Autodesk Inventor part; units mm, degrees
ref_plane "YZ Plane" through (0, 0, 0) normal (1, 0, 0) x (0, 1, 0)
ref_plane "XZ Plane" through (0, 0, 0) normal (0, 1, 0) x (-1, 0, 0)
ref_plane "XY Plane" through (0, 0, 0) normal (0, 0, 1) x (1, 0, 0)
sketch "Sketch1" plane through (0, 0, 0) normal (0, 1, 0) x (-1, 0, 0)
  line L0 (0, 780) -> (0, 0)
  line L1 (727.158, 778) -> (727.158, 780)
  line L2 (727.158, 780) -> (0, 780)
  line L3 (727.158, 778) -> (110, 0)
  line L4 (110, 0) -> (0, 0)
  point P0 (0, 678)
  dimension "d1" = 727.158
  dimension "d2" = 2
  dimension "d5" = 128.424
  dimension "d6" = 110
  dimension "d9" = 780
extrude "Plate1" add sketch "Sketch1" along normal blind 3
mirror "Mirror1" about plane through (0, 0, 0) normal (1, 0, 0)
sketch "Sketch2" plane through (0, 0, 0) normal (0, -1, 0) x (1, 0, 0)
  line L0 (-110, 0) -> (110, 0) construction
  line L1 (-110, 0) -> (-727.158, 778) construction
  circle A0 centre (-325, 450) radius 84.5
  line L2 (110, 0) -> (727.158, 778) construction
  circle A1 centre (100, 450) radius 84.5
  circle A2 centre (410, 600) radius 45
  line L3 (-110, 0) -> (110, 0) construction
  line L4 (-240.5, 450) -> (-240.5, 164.5105) construction
  line L5 (365, 600) -> (365, 0) construction
  line L6 (-325, 534.5) -> (365, 534.5) construction
  line L7 (-325, 365.5) -> (365, 365.5) construction
  line L8 (100, 534.5) -> (365, 534.5) construction
  line L9 (410, 555) -> (365, 555) construction
  line L10 (-727.158, 780) -> (727.158, 780)
  line L11 (-727.158, 778) -> (-727.158, 780)
  line L12 (727.158, 778) -> (727.158, 780)
  point P0 (0, 0)
  point P1 (0, 0)
  point P2 (0, 0)
  point P3 (0, 0)
  point P4 (0, 0)
  point P5 (0, 0)
  point P6 (0, 0)
  dimension "d13" = 169
  dimension "d16" = 450
  dimension "d17" = 450
  dimension "d18" = 325
  dimension "d19" = -169
  dimension "d20" = 90
  dimension "d23" = 410
  dimension "d24" = 600
  dimension "d29" = 100
extrude "Extrusion1" cut sketch "Sketch2" against normal through all
sketch "Sketch3" plane through (0, 0, 0) normal (0, -1, 0) x (1, 0, 0)
  line L0 (-53.9958, 701.8167) -> (-53.9958, 713.8167) construction
  line L1 (-53.9958, 713.8167) -> (56.0042, 713.8167) construction
  line L2 (56.0042, 713.8167) -> (56.0042, 701.8167) construction
  line L3 (56.0042, 701.8167) -> (-53.9958, 701.8167) construction
  point P0 (0, 0)
  point P1 (1.0042, 701.8167)
  dimension "d25" = 12
  dimension "d26" = 110
mark "Mark1"
equation "\"d3\" = Thickness"
properties part number "MSC 701 FACE 1" material "Stainless Steel"
The listing builds one solid part. Answer for the finished solid, in the listing's coordinates (mm). Round coordinates to 2 decimals unless told otherwise and drop trailing zeros. Write each loop counter-clockwise with the first axis right and the second up, starting at its lowest first coordinate (ties: lowest second). Pieces come first, ordered by that corner, then holes. Notation, with made-up numbers: (-34.5, 38.25) -> (-26.5, 38.25) arc R12 ccw to (-26.5, 47.25) -> close; hole circle Ø8 at (37, 76). An arc over 180 degrees is marked (long way). Answer as a JSON object with one key per item and string values. Group by question number.
Q1. This flat-tipped pin is pushed along its axis until it touches: pin 1 Ø1 at (x, y) = (461, 2) entering from -Z. Where does it stop, or does it pass through?
Q2. Straight lines are drawn through the part: line 1 along X through (y, z) = (0.1, 498); line 2 along Z through (x, y) = (178, 1.95); line 3 along Z through (x, y) = (-325, 1.6). For each, find the intervals that lie inside material, in ascending order.
Q3. Section D-D (z = 450) is taken. Write down the section's boundary in (x, y).
Q4. Section A-A (z = 619) is taken. Write down the section's boundary in (x, y), plus the area to 3 significant figures.
Q5. Section C-C (y = 2.3) is taken. Write down the section's boundary in (x, z), plus the area to 3 significant figures.
Q6. Section B-B (x = -325) is taken. Write down the section's boundary in (y, z), plus the area to 3 significant figures.
Q7. Determine the mould class of faces 1 (the face through (434.192, 1.479, 637.944)), 2 (the face through (10, 3, 482)), 3 (the face through (-246.94, 1.48, 417.64)), 4 (the face through (414.259, 1.479, 383.554)) for opening direction Z: pulls with the +Z half, pulls with the -Z half, needs draft (parallel to the pull), parting line crosses it, or undercut.
Check values:
{
 "1": {"pin 1": "z = 441.85"},
 "2": {"line 1": "-505.04 to -394.54, -255.46 to 30.46, 169.54 to 505.04", "line 2": "85.72 to 417.5, 482.5 to 780", "line 3": "271.03 to 365.5, 534.5 to 780"},
 "3": {"outline": "(-466.97, 0) -> (-409.5, 0) -> (-409.5, 3) -> (-466.97, 3) -> close; (-240.5, 0) -> (15.5, 0) -> (15.5, 3) -> (-240.5, 3) -> close; (184.5, 0) -> (466.97, 0) -> (466.97, 3) -> (184.5, 3) -> close"},
 "4": {"outline": "(-601.03, 0) -> (369.21, 0) -> (369.21, 3) -> (-601.03, 3) -> close; (450.79, 0) -> (601.03, 0) -> (601.03, 3) -> (450.79, 3) -> close", "area": "3,360 mm^2"},
 "5": {"outline": "(-727.16, 778) -> (-110, 0) -> (110, 0) -> (727.16, 778) -> (727.16, 780) -> (-727.16, 780) -> close; hole circle Ø169 at (-325, 450); hole circle Ø169 at (100, 450); hole circle Ø90 at (410, 600)", "area": "603,000 mm^2"},
 "6": {"outline": "(0, 271.03) -> (3, 271.03) -> (3, 365.5) -> (0, 365.5) -> close; (0, 534.5) -> (3, 534.5) -> (3, 780) -> (0, 780) -> close", "area": "1,020 mm^2"},
 "7": {"face 1": "undercut", "face 2": "needs draft", "face 3": "undercut", "face 4": "pulls with the -Z half"}
}
